```python
from build123d import *

# Parameters (mm, degrees)
SKETCH1_R            = 0.79375
EXTRUDE1_DEPTH       = 1.5875
FILLET2_R            = 0.508
SKETCH2_R            = 0.79375
EXTRUDE2_DEPTH       = 1.27
CUT_EXTRUDE1_DEPTH   = 1.0795
MIRROR2_COPY_1_DEPTH = 1.0795


with BuildPart() as part:
    # Sketch1 → Extrude1 (new body)
    with BuildSketch(Plane(origin=(0, 0, 0), x_dir=(1, 0, 0), z_dir=(0, 1, 0))):
        with BuildLine():
            Line((-18.6055, 9.8425), (18.6055, 9.8425))
            ThreePointArc((18.6055, 9.8425), (19.144315367, 9.619315367), (19.3675, 9.0805))
            Line((19.3675, 9.0805), (19.3675, -9.0805))
            ThreePointArc((19.3675, -9.0805), (19.144315367, -9.619315367), (18.6055, -9.8425))
            Line((18.6055, -9.8425), (-18.6055, -9.8425))
            ThreePointArc((-18.6055, -9.8425), (-19.144315367, -9.619315367), (-19.3675, -9.0805))
            Line((-19.3675, -9.0805), (-19.3675, 9.0805))
            ThreePointArc((-19.3675, 9.0805), (-19.144315367, 9.619315367), (-18.6055, 9.8425))
        make_face()
        with Locations((-17.3355, 7.8105)):
            Circle(SKETCH1_R, mode=Mode.SUBTRACT)
        with Locations((17.3355, 7.8105)):
            Circle(SKETCH1_R, mode=Mode.SUBTRACT)
        with Locations((17.3355, -7.8105)):
            Circle(SKETCH1_R, mode=Mode.SUBTRACT)
        with Locations((-17.3355, -7.8105)):
            Circle(SKETCH1_R, mode=Mode.SUBTRACT)
    extrude(amount=EXTRUDE1_DEPTH)

    # Fillet2
    fillet2_edges = [part.edges().sort_by_distance(p)[0] for p in [
        (-19.3675, 0, 0),
        (-19.144315367, 0, -9.619315367),
        (0, 0, -9.8425),
        (19.144315367, 0, -9.619315367),
        (19.3675, 0, 0),
        (19.144315367, 0, 9.619315367),
        (0, 0, 9.8425),
        (-19.144315367, 0, 9.619315367),
    ]]
    fillet(fillet2_edges, radius=FILLET2_R)

    # Sketch2 → Extrude2 (add)
    with BuildSketch(Plane(origin=(0, 1.5875, 0), x_dir=(-1, 0, 0), z_dir=(0, 1, 0))):
        with BuildLine():
            Line((18.6055, 9.2075), (-18.6055, 9.2075))
            ThreePointArc((-18.6055, 9.2075), (-18.695302561, 9.170302561), (-18.7325, 9.0805))
            Line((-18.7325, 9.0805), (-18.7325, -9.0805))
            ThreePointArc((-18.7325, -9.0805), (-18.695302561, -9.170302561), (-18.6055, -9.2075))
            Line((-18.6055, -9.2075), (18.6055, -9.2075))
            ThreePointArc((18.6055, -9.2075), (18.695302561, -9.170302561), (18.7325, -9.0805))
            Line((18.7325, -9.0805), (18.7325, 9.0805))
            ThreePointArc((18.7325, 9.0805), (18.695302561, 9.170302561), (18.6055, 9.2075))
        make_face()
        with Locations((-17.3355, 7.8105)):
            Circle(SKETCH2_R, mode=Mode.SUBTRACT)
        with Locations((-17.3355, -7.8105)):
            Circle(SKETCH2_R, mode=Mode.SUBTRACT)
        with Locations((17.3355, -7.8105)):
            Circle(SKETCH2_R, mode=Mode.SUBTRACT)
        with Locations((17.3355, 7.8105)):
            Circle(SKETCH2_R, mode=Mode.SUBTRACT)
        with BuildLine():
            Line((-18.6055, -7.228512887), (-18.6055, 7.228512887))
            ThreePointArc((-18.6055, 7.228512887), (-16.347671827, 6.822671827), (-16.753512887, 9.0805))
            Line((-16.753512887, 9.0805), (16.753512887, 9.0805))
            ThreePointArc((16.753512887, 9.0805), (16.347671827, 6.822671827), (18.6055, 7.228512887))
            Line((18.6055, 7.228512887), (18.6055, -7.228512887))
            ThreePointArc((18.6055, -7.228512887), (16.347671827, -6.822671827), (16.753512887, -9.0805))
            Line((16.753512887, -9.0805), (-16.753512887, -9.0805))
            ThreePointArc((-16.753512887, -9.0805), (-16.347671827, -6.822671827), (-18.6055, -7.228512887))
        make_face(mode=Mode.SUBTRACT)
    extrude(amount=EXTRUDE2_DEPTH)

    # Sketch3 → Cut-Extrude1 (cut)
    with BuildSketch(Plane.XZ):
        with BuildLine():
            Line((-16.3195, -5.5245), (-19.3675, -5.5245))
            Line((-19.3675, -5.5245), (-19.3675, -9.8425))
            Line((-19.3675, -9.8425), (-15.0495, -9.8425))
            Line((-15.0495, -9.8425), (-15.0495, -6.7945))
            ThreePointArc((-15.0495, -6.7945), (-15.421474388, -5.896474388), (-16.3195, -5.5245))
        make_face()
    cut_extrude1 = extrude(amount=-CUT_EXTRUDE1_DEPTH, mode=Mode.SUBTRACT)

    # Mirror1: Cut-Extrude1 across plane
    add(cut_extrude1.mirror(Plane(origin=(0, 0, 0), x_dir=(0, 0, 1), z_dir=(1, 0, 0))), mode=Mode.SUBTRACT)

    # Mirror2: Cut-Extrude1 across plane
    add(cut_extrude1.mirror(Plane.XY), mode=Mode.SUBTRACT)

    # Mirror2 copy 1 sketch → Mirror2 copy 1 (cut)
    with BuildSketch(Plane(origin=(0, 0, 0), x_dir=(-1, 0, 0), z_dir=(0, -1, 0))):
        with BuildLine():
            Line((-16.3195, -5.5245), (-19.3675, -5.5245))
            Line((-19.3675, -5.5245), (-19.3675, -9.8425))
            Line((-19.3675, -9.8425), (-15.0495, -9.8425))
            Line((-15.0495, -9.8425), (-15.0495, -6.7945))
            ThreePointArc((-15.0495, -6.7945), (-15.421474388, -5.896474388), (-16.3195, -5.5245))
        make_face()
    extrude(amount=-MIRROR2_COPY_1_DEPTH, mode=Mode.SUBTRACT)


solid = part.part
```
Read the model definition and answer for the solid it produces. Units are mm, in the model's axes. A direction names the side the tool comes from. Give positions to 0.01 mm unless a question says otherwise; leave off trailing zeros. Loops run counter-clockwise (first coordinate to the right, second up) from the corner with the lowest first, then second, coordinate; pieces in that order, holes last.
Item 1: Find the intervals of material crossed by line 1 along X through (y, z) = (1.25, 7.75); line 2 along X through (y, z) = (2.4, 8.25); line 3 along Y through (x, z) = (2, 2.25), in increasing order.
Item 2: The mould has two halves that part along Z. Classify faces 6 (the flat face through (0, 0, 0)), 7 (the cylindrical face through (16.37, 2.21, 6.8)), 8 (the flat face through (0, 1.588, 0)), 9 (the cylindrical face through (-15.41, 0.53, -5.91)): released by +Z, released by -Z, zero draft, split by the parting line, or undercut.
Item 3: The part is cut by section D-D (x = -15.5). Write down the section's boundary in (y, z), and give its area (3 significant figures).
Item 4: The part is cut by section A-A (x = 5). Write down the section's boundary in (y, z), and give its area (3 significant figures).
Item 5: Each of these flat-tipped pins is pushed along its axis until it touches: pin 1 Ø1.3 at (x, z) = (16.5, 8) entering from -Y; pin 2 Ø0.5 at (y, z) = (0.5, -9) entering from -X; pin 3 Ø1.4 at (y, z) = (2.5, -0.5) entering from +X. Where does it stop, or does it pass through?
Item 6: For faces 1 (the flat face through (-17.8, 0.5, -5.524)), 2 (the flat face through (15.05, 0.5, 8.3)), 3 (the flat face through (-17.8, 0.5, 5.524)), 4 (the flat face through (19.368, 1, 0)), 5 (the cylindrical face through (15.41, 0.53, -5.91)), determine the directions among +Z, -Z, +X, -X, +Y, -Y from which every point of the face is accessible in a straight line to the end or side of a thin tool.
Item 7: The part is cut by section C-C (z = 0.5). Write down the section's boundary in (x, y).
Item 8: The part is cut by section B-B (y = 2.3). Write down the section's boundary in (x, z), and give its area (3 significant figures).
Taken from the geometry:
1. line 1: x = -19.37 to -18.13, -16.54 to 16.54, 18.13 to 19.37
1. line 2: x = -18.73 to -18, -16.67 to -16.01, 16.01 to 16.67, 18 to 18.73
1. line 3: y = 0 to 1.59
2. face 6: zero draft
2. face 7: undercut
2. face 8: undercut
2. face 9: released by -Z
3. outline: (0, -5.82) - (1.08, -5.82) - (1.08, -9.84) - (1.59, -9.84) - (1.59, -9.21) - (2.86, -9.21) - (2.86, -9.08) - (1.59, -9.08) - (1.59, 9.08) - (2.86, 9.08) - (2.86, 9.21) - (1.59, 9.21) - (1.59, 9.84) - (1.08, 9.84) - (1.08, 5.82) - (0, 5.82) - close
3. area: 22.9 mm2
4. outline: (0, -9.33) arc R0.51 ccw to (0.51, -9.84) - (1.59, -9.84) - (1.59, -9.21) - (2.86, -9.21) - (2.86, -9.08) - (1.59, -9.08) - (1.59, 9.08) - (2.86, 9.08) - (2.86, 9.21) - (1.59, 9.21) - (1.59, 9.84) - (0.51, 9.84) arc R0.51 ccw to (0, 9.33) - close
4. area: 31.5 mm2
5. pin 1: stops at y = 1.08
5. pin 2: stops at x = -15.05
5. pin 3: stops at x = 18.73
6. face 1: -Z, -X, -Y
6. face 2: +Z, +X, -Y
6. face 3: +Z, -X, -Y
6. face 4: +Z, -Z, +X, +Y, -Y
6. face 5: -Z, +X, -Y
7. outline: (-19.37, 0.51) arc R0.51 ccw to (-18.86, 0) - (18.86, 0) arc R0.51 ccw to (19.37, 0.51) - (19.37, 1.59) - (18.73, 1.59) - (18.73, 2.86) - (18.61, 2.86) - (18.61, 1.59) - (-18.61, 1.59) - (-18.61, 2.86) - (-18.73, 2.86) - (-18.73, 1.59) - (-19.37, 1.59) - close
8. outline: (-18.73, -9.08) arc R0.13 ccw to (-18.61, -9.21) - (18.61, -9.21) arc R0.13 ccw to (18.73, -9.08) - (18.73, 9.08) arc R0.13 ccw to (18.61, 9.21) - (-18.61, 9.21) arc R0.13 ccw to (-18.73, 9.08) - close; hole (-18.61, -7.23) arc R1.4 cw (long way) to (-16.75, -9.08) - (16.75, -9.08) arc R1.4 cw (long way) to (18.61, -7.23) - (18.61, 7.23) arc R1.4 cw (long way) to (16.75, 9.08) - (-16.75, 9.08) arc R1.4 cw (long way) to (-18.61, 7.23) - close; hole circle Ø1.59 at (-17.34, -7.81); hole circle Ø1.59 at (-17.34, 7.81); hole circle Ø1.59 at (17.34, -7.81); hole circle Ø1.59 at (17.34, 7.81)
8. area: 30.6 mm2
